Build history of the part. All positions in model axes, mm. A direction names the side the tool comes from. Give positions to 0.01 mm unless a question says otherwise; leave off trailing zeros. Order: outer loops, then holes, each group sorted by start corner. A loop starts at its lowest first (then second) coordinate and runs counter-clockwise, first axis right, second up. Notation, with made-up numbers: (58, -24) - (108, -24) arc R27 cw to (108, -2) - close; hole circle Ø2 at (-23, 42). An arc over 180 degrees is marked (long way). One line per item, written item: value.
```python
from build123d import *

# Parameters (mm, degrees)
F1_DEPTH       = 19.05
F3_D           = 3.175
F3_CSINK_D     = 6.35
F3_CSINK_ANGLE = 90
F5_D           = 17.78
F7_DEPTH       = 38.101
F8_R           = 5.08
F9_R           = 5.08


with BuildPart() as f1:
    # F0 (on Right) → F1 (new body, symmetric)
    with BuildSketch(Plane.YZ):
        Polygon((4.68586, 25.4), (0, 25.4), (0, 0), (38.1, 0), (38.1, 4.68586), (4.68586, 4.68586), align=None)
    extrude(amount=F1_DEPTH, both=True)

    # F3 (through all)
    with Locations(Plane(origin=(0, 4.68586, 0), x_dir=(-1, 0, 0), z_dir=(0, 1, 0))):
        with Locations((0, 20.114239)):
            CounterSinkHole(F3_D / 2, F3_CSINK_D / 2, counter_sink_angle=F3_CSINK_ANGLE)

    # F5 (through all)
    with Locations(Plane.XY.offset(4.68586)):
        with Locations((0, 21.39293)):
            Hole(F5_D / 2)

    # F6 (on face) → F7 (cut, through all)
    with BuildSketch(Plane.YZ.offset(19.05)):
        with BuildLine():
            Line((25.20293, 4.68586), (17.58293, 4.68586))
            ThreePointArc((17.58293, 4.68586), (21.39293, 0.87586), (25.20293, 4.68586))
        make_face()
    extrude(amount=-F7_DEPTH, mode=Mode.SUBTRACT)

    # F8
    f8_edges = [f1.edges().sort_by_distance(p)[0] for p in [
        (0, 4.68586, 4.68586),
    ]]
    fillet(f8_edges, radius=F8_R)

    # F9
    f9_edges = [f1.edges().sort_by_distance(p)[0] for p in [
        (19.05, 38.1, 2.34293),
        (-19.05, 38.1, 2.34293),
        (19.05, 2.34293, 25.4),
        (-19.05, 2.34293, 25.4),
    ]]
    fillet(f9_edges, radius=F9_R)


solid = f1.part
```
(1) Pin check, flat tips, straight feed: P1, Ø1, axis at x = 0, z = 7.5, coming from the +Y side; P2, Ø6, axis at x = -0.5, y = 32, coming from the +Z side; P3, Ø5, axis at x = 3, y = 10, coming from the -Z side; P4, Ø4.5, axis at x = 2, z = 18.5, coming from the +Y side. Stop position of each tip, or through.
Completed:
P1: y = 5.5
P2: z = 4.69
P3: z = 0
P4: y = 4.69
(2) Slice it at B-B, the plane y = 16. Give the cut face in (x, z).
Completed:
outline: (-19.05, 0) - (-7.07, 0) - (-7.07, 4.69) - (-19.05, 4.69) - close; (7.07, 0) - (19.05, 0) - (19.05, 4.69) - (7.07, 4.69) - close
(3) 3-axis set-ups, long thin cutter, end or side, ignore diameter. For faces 4 (the face through (17.522, 2.31, 23.951)), 5 (the face through (0, 32, 4.686)): which of +Z, -Z, +X, -X, +Y, -Y reach the whole face in a straight line?
Completed:
face 4: +Z, +X, +Y, -Y
face 5: +Z, +X, -X, +Y
(4) Slice it at C-C, the plane x = 10.5. Give the cut face in (y, z).
Completed:
outline: (0, 0) - (38.1, 0) - (38.1, 4.69) - (25.2, 4.69) arc R3.81 cw to (17.58, 4.69) - (9.77, 4.69) arc R5.08 cw to (4.69, 9.77) - (4.69, 25.4) - (0, 25.4) - close
(5) Slice it at A-A, the plane x = 0. Give the cut face in (y, z).
Completed:
outline: (0, 0) - (12.5, 0) - (12.5, 4.69) - (9.77, 4.69) arc R5.08 cw to (4.69, 9.77) - (4.69, 16.94) - (3.1, 18.53) - (0, 18.53) - close; (0, 21.7) - (3.1, 21.7) - (4.69, 23.29) - (4.69, 25.4) - (0, 25.4) - close; (30.28, 0) - (38.1, 0) - (38.1, 4.69) - (30.28, 4.69) - close
(6) Drill centre lines: line 1 (Y direction, x = 0, z = 2.3); line 2 (Z direction, x = 0, y = 1.35); line 3 (Z direction, x = 11, y = 17.5). Where is each one in solid material? Low to high.
Completed:
line 1: 0 to 12.5, 30.28 to 38.1
line 2: 0 to 18.53, 21.7 to 25.4
line 3: 0 to 4.69
(7) Pull direction Y, two halves, no side cores. Call faces 1 (the face through (0, 12, 4.686)), 2 (the face through (7.05, 15.98, 2.31)), 3 (the face through (-17.601, 36.572, 2.376)): +Y half, -Y half, draft (parallel to the pull), parting line (faces both ways), or undercut.
Completed:
face 1: draft
face 2: undercut
face 3: +Y half
(8) Slice it at D-D, the plane y = 11. Give the cut face in (x, z).
Completed:
outline: (-19.05, 0) - (19.05, 0) - (19.05, 4.69) - (-19.05, 4.69) - close
